Here's the drawing with two shaded views (mm, measured from the low corner). I have some questions. A direction names the side the tool comes from. Round coordinates to 2 decimals unless told otherwise and drop trailing zeros. Loops run counter-clockwise (first coordinate to the right, second up) from the corner with the lowest first, then second, coordinate; pieces in that order, holes last. Notation, with made-up numbers: M 86,-6.5 L 99,-6.5 A10 ccw 99,0.5 Z; hole C 6,53.25 d9. An arc over 180 degrees is marked long. Answer as CSV lines item,"result".
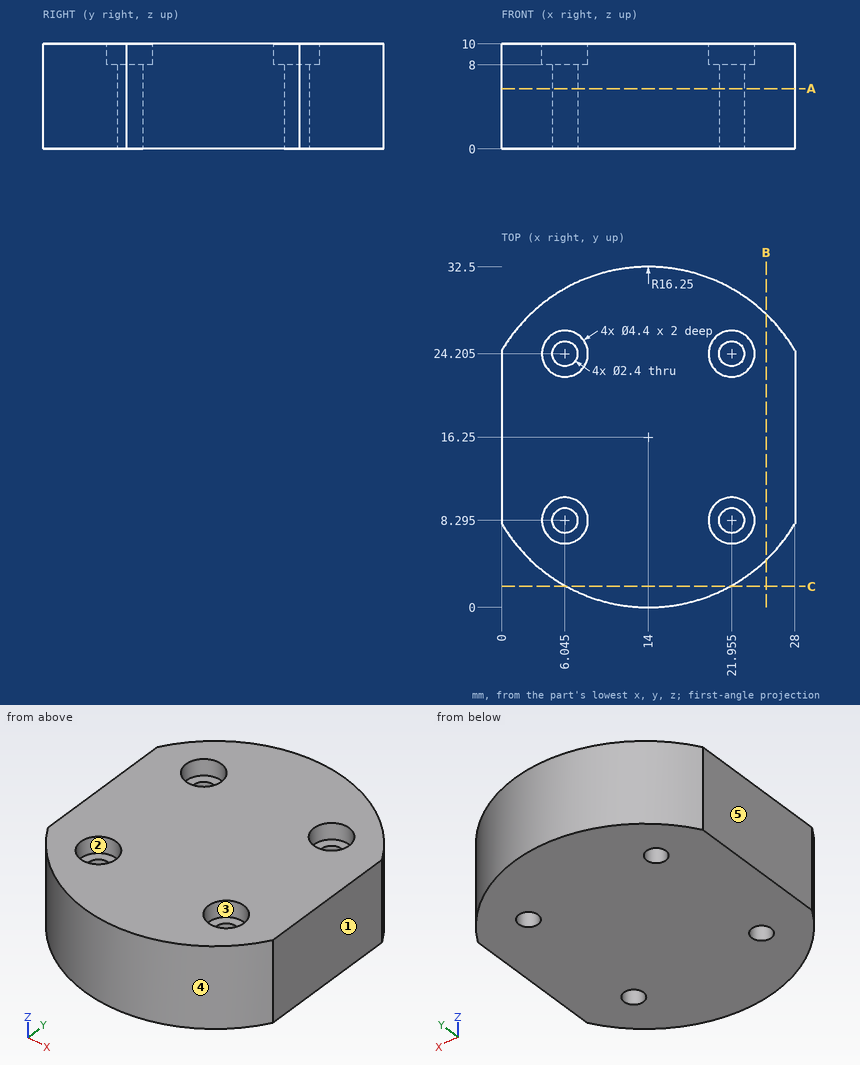
1. We'd pull the mould along Y, two halves only. Please class the marked faces 3, 4 and 5: pulls with the +Y half, pulls with the -Y half, needs draft (parallel to the pull), parting line crosses it, or undercut.
Evaluation:
face 3,"undercut"
face 4,"pulls with the -Y half"
face 5,"needs draft"
2. I want a section at C-C, the plane y = 2. Please give me the cut outline in (x, z).
Evaluation:
outline,"M 6.19,0 L 21.81,0 L 21.81,10 L 6.19,10 Z"
3. Which directions (+Z, -Z, +X, -X, +Y, -Y) give clear straight access to the entire face, cutting with the end or side of a thin tool? Please do the marked faces 1 and 2.
Evaluation:
face 1,"+Z, -Z, +X, +Y, -Y"
face 2,"+Z"
4. For P1, Ø1.3, axis at x = 5, y = 8.5, coming from the +Z side; P2, Ø2, axis at y = 26, z = 2.5, coming from the -X side; P3, Ø1, axis at y = 5.5, z = 2.5, coming from the -X side, each with a flat end and sliding along its axis, tell me the tip position at first contact or that it passes through.
Evaluation:
P1,"stops at z = 8"
P2,"stops at x = 0.31"
P3,"stops at x = 1.39"
5. I want a section at A-A, the plane z = 5.75. Please give me the cut outline in (x, y) (3 decimals).
Evaluation:
outline,"M 0,8 A16.25 ccw 28,8 L 28,24.5 A16.25 ccw 0,24.5 Z; hole C 6.045,8.295 d2.4; hole C 6.045,24.205 d2.4; hole C 21.955,8.295 d2.4; hole C 21.955,24.205 d2.4"
6. I want a section at B-B, the plane x = 25.25. Please give me the cut outline in (y, z).
Evaluation:
outline,"M 4.52,0 L 27.98,0 L 27.98,10 L 4.52,10 Z"
7. If I drill on line 1 (Y direction, x = 23.25, z = 9.5); line 2 (Y direction, x = 5, z = 7) (1 decimal); line 3 (Z direction, x = 22.75, y = 23), over which ranges is the centre line in solid material (lowest first)? Write a range as [from, to].
Evaluation:
line 1,"y = [2.89, 6.52], [10.07, 22.43], [25.98, 29.61]"
line 2,"y = [2.7, 7.7], [8.9, 23.6], [24.8, 29.8]"
line 3,"z = [0, 8]"
